from build123d import *

# Parameters (mm, degrees)
SKETCH_1_R      = 8
EXTRUDE_3_DEPTH = 25
SKETCH_3_R      = 10
EXTRUDE_4_DEPTH = 3
EXTRUDE_START   = 3
SKETCH_4_R      = 10
EXTRUDE_5_DEPTH = 3


with BuildPart() as part:
    # 草图1 → 凸台-拉伸3 (new body)
    with BuildSketch(Plane.XY):
        Circle(SKETCH_1_R)
    extrude(amount=EXTRUDE_3_DEPTH)

    # 草图3 → 凸台-拉伸4 (add)
    with BuildSketch(Plane.XY.offset(25)):
        Circle(SKETCH_3_R)
    extrude(amount=EXTRUDE_4_DEPTH)

    # 草图4 → 凸台-拉伸5 (add)
    with BuildSketch(Plane(origin=(0, 0, 0), x_dir=(-1, 0, 0), z_dir=(0, 0, -1)).offset(EXTRUDE_START)):
        with Locations(Location((0, 0, 0), (0, 0, 180))):
            Circle(SKETCH_4_R)
    extrude(amount=-EXTRUDE_5_DEPTH)


solid = part.part
The listing builds one solid part. Answer for the finished solid, in the listing's coordinates (mm). A direction names the side the tool comes from. Give positions to 0.01 mm unless a question says otherwise; leave off trailing zeros. Loops run counter-clockwise (first coordinate to the right, second up) from the corner with the lowest first, then second, coordinate; pieces in that order, holes last. Notation, with made-up numbers: (-21, 3.5) - (36, 3.5) arc R27 cw to (36, 42.5) - close; hole circle Ø3 at (9, 13.25). An arc over 180 degrees is marked (long way). Write each question's results on one line, items separated by ' | '.
1. Find section C-C, the plane y = -8.5. Write down the section's boundary in (x, z).
Resolved:
outline: (-5.27, -3) - (5.27, -3) - (5.27, 0) - (-5.27, 0) - close; (-5.27, 25) - (5.27, 25) - (5.27, 28) - (-5.27, 28) - close
2. Which of the six approach directions +Z, -Z, +X, -X, +Y, -Y give full straight-line access (tool end or side, diameter ignored) to faces 4 (the face through (-2.17, -9.76, 26.48)), 5 (the face through (-1.73, -7.81, 12.32))?
Resolved:
face 4: +Z, -Z | face 5: none
3. Find section D-D, the plane z = 5. Write down the section's boundary in (x, y).
Resolved:
outline: circle Ø16 at (0, 0)
4. For a pull along Z with two mould halves and no side action, classify faces 1 (the face through (0, 8.2, 25)), 2 (the face through (-10, 0, -2)), 3 (the face through (0, 0, -3)) as +Z half, -Z half, draft (parallel to the pull), parting line (faces both ways), or undercut.
Resolved:
face 1: undercut | face 2: draft | face 3: -Z half
5. Find section A-A, the plane y = 0. Write down the section's boundary in (x, z), then the cut area to 3 significant figures.
Resolved:
outline: (-10, -3) - (10, -3) - (10, 0) - (8, 0) - (8, 25) - (10, 25) - (10, 28) - (-10, 28) - (-10, 25) - (-8, 25) - (-8, 0) - (-10, 0) - close | area: 520 mm^2
6. Flat-ended cylindrical pins translate along their axes: P1, Ø5, axis at x = -7.5, z = 22, coming from the +Y side (3 decimals); P2, Ø8, axis at y = -6.5, z = 6, coming from the -X side; P3, Ø1.5, axis at y = 0.5, z = 17.5, coming from the +X side. Find the tip coordinate at first contact, or state that the pin passes through.
Resolved:
P1: stops at y = 6.245 | P2: stops at x = -7.6 | P3: stops at x = 8
7. Consider probe 1 along Z at (x, y) = (-4.25, 9); probe 2 along Y at (x, z) = (0, 1); probe 3 along Y at (x, z) = (6.75, 3). Determine where each line is inside the solid, lowest interval first. Write a range as from..to.
Resolved:
probe 1: z = -3..0, 25..28 | probe 2: y = -8..8 | probe 3: y = -4.29..4.29
